Could you check a few things on this model? Use its own coordinates, in mm. A direction names the side the tool comes from. Coordinates: 2 decimals unless noted, no trailing zeros. Order: outer loops, then holes, each group sorted by start corner. A loop starts at its lowest first (then second) coordinate and runs counter-clockwise, first axis right, second up. Notation, with made-up numbers: (28.5, 8.25) - (56.5, 8.25) arc R24 ccw to (56.5, 22.25) - close; hole circle Ø11 at (76.25, 58.5). An arc over 180 degrees is marked (long way). Answer as a JSON object with one key per item and string values. Group by question number.
(1) We'd pull the mould along Z, two halves only. Please class faces 1 (the flat face through (-111.584, 11.826, 12.167)), 2 (the flat face through (-113, 10, 63.5)), 3 (the flat face through (-189, 17, 63.5)): pulls with the +Z half, pulls with the -Z half, needs draft (parallel to the pull), parting line crosses it, or undercut.
(2) Imagine slicing it at A-A, the plane z = 39.5. Give the number of separate pieces and of enclosed holes in the cut face, and give its area (3 significant figures).
(3) Which directions (+Z, -Z, +X, -X, +Y, -Y) give clear straight access to the entire face, cutting with the end or side of a thin tool? Please do faces 4 (the flat face through (-108.49, 8.38, 12.17)), 5 (the flat face through (-6, 3.175, 38)).
(4) Imagine slicing it at B-B, the plane x = -6.35. Write out the boundary of the cut face in (y, z) (3 decimals), and give its area (3 significant figures).
(5) Imagine slicing it at C-C, the plane x = -191. Write out the boundary of the cut face in (y, z).
(6) Will these pins go through, and if not, where does the flat tip stop? P1, Ø3, axis at x = -6.35, z = 63.5, coming from the -Y side; P2, Ø4.5, axis at x = -64, y = 6.5, coming from the -Z side; P3, Ø6.5, axis at x = -6.5, z = 22.5, coming from the +Y side (3 decimals); P4, Ø2, axis at x = -155, z = 48, coming from the +Y side.
(7) Please list where these lines run through material, in increasing order: probe 1 along Z at (x, y) = (-6.35, 1.4); probe 2 along Z at (x, y) = (-162.5, 15); probe 3 along Y at (x, z) = (-12.5, 36) (3 decimals).
from build123d import *

# Parameters (mm, degrees)
BOSS_EXTRUDE1_DEPTH = 76.2
SKETCH2_R           = 1.778
CUT_EXTRUDE1_DEPTH  = 76.2
SKETCH3_W           = 12.7
SKETCH3_H           = 50.8
CUT_EXTRUDE2_DEPTH  = 76.2
LPATTERN1_COUNT     = 7
LPATTERN1_PITCH     = 25.4


with BuildPart() as part:
    # Sketch1 → Boss-Extrude1 (new body)
    with BuildSketch(Plane.XY):
        Polygon((0, 0), (-12.7, 0), (-207.009499064, 16.999878384), (-207.737954037, 20.238609936), (-12.7, 3.175), (0, 3.175), align=None)
    extrude(amount=BOSS_EXTRUDE1_DEPTH)

    # Sketch2 → Cut-Extrude1 (cut)
    with BuildSketch(Plane(origin=(0, 3.175, 0), x_dir=(1, 0, 0), z_dir=(0, 1, 0))):
        with Locations((-6.35, -12.7)):
            Circle(SKETCH2_R)
        with Locations((-6.35, -63.5)):
            Circle(SKETCH2_R)
    extrude(amount=-CUT_EXTRUDE1_DEPTH, mode=Mode.SUBTRACT)

    # Sketch3 → Cut-Extrude2 (cut)
    with BuildSketch(Plane(origin=(0.179195714, 2.04821638, 0), x_dir=(0.996194698, -0.087155743, 0), z_dir=(0.087155743, 0.996194698, 0))):
        with Locations((-189.661359485, -38.1)):
            Rectangle(SKETCH3_W, SKETCH3_H)
    cut_extrude2 = extrude(amount=-CUT_EXTRUDE2_DEPTH, mode=Mode.SUBTRACT)

    # LPattern1: Cut-Extrude2 ×7
    with Locations(*[Vector(0.996194698, -0.087155743, 0) * (i * LPATTERN1_PITCH) for i in range(1, LPATTERN1_COUNT)]):
        add(cut_extrude2, mode=Mode.SUBTRACT)


solid = part.part
Result set:
{
 "1": {"face 1": "needs draft", "face 2": "undercut", "face 3": "undercut"},
 "2": {"separate pieces": "8", "enclosed holes": "0", "area": "377 mm^2"},
 "3": {"face 4": "+Z, -Z, -X, -Y", "face 5": "+Z, -Z, +X, +Y"},
 "4": {"outline": "(0, 0) - (3.175, 0) - (3.175, 10.922) - (0, 10.922) - close; (0, 14.478) - (3.175, 14.478) - (3.175, 61.722) - (0, 61.722) - close; (0, 65.278) - (3.175, 65.278) - (3.175, 76.2) - (0, 76.2) - close", "area": "219 mm^2"},
 "5": {"outline": "(15.6, 0) - (18.77, 0) - (18.77, 12.7) - (15.6, 12.7) - close; (15.6, 63.5) - (18.77, 63.5) - (18.77, 76.2) - (15.6, 76.2) - close"},
 "6": {"P1": "passes through", "P2": "stops at z = 0", "P3": "stops at y = 3.175", "P4": "stops at y = 15.71"},
 "7": {"probe 1": "z = 0 to 10.92, 14.48 to 61.72, 65.28 to 76.2", "probe 2": "z = 0 to 12.7, 63.5 to 76.2", "probe 3": "y = 0 to 3.175"}
}
